Autodesk Inventor part; units mm, degrees
ref_plane "Plano de trabajo1" through (0, 5, -50) normal (1, 0, 0) x (0, 0, -1)
ref_plane "Plano de trabajo2" through (0, 15, 0) normal (0, -1, 0) x (1, 0, 0)
ref_plane "YZ Plane" through (0, 0, 0) normal (1, 0, 0) x (0, 1, 0)
sketch "Boceto1" plane through (0, 0, 0) normal (0, 1, 0) x (-1, 0, 0)
  line L0 (27.5, 50) -> (-27.5, 50)
  line L1 (-27.5, 50) -> (-27.5, -50)
  line L2 (-27.5, -50) -> (27.5, -50)
  line L3 (27.5, -50) -> (27.5, 50)
  line L4 (27.5, 50) -> (-27.5, -50) construction
  line L5 (-27.5, 50) -> (27.5, -50) construction
  point P0 (0, 0)
  dimension "d0" = 55
  dimension "d1" = 100
extrude "Extrusión1" add sketch "Boceto1" along normal blind 30
sketch "Boceto2" plane through (27.5, 0, -50) normal (0, 0, -1) x (-1, 0, 0)
  line L0 (22.5, 25) -> (32.5, 25)
  line L1 (32.5, 25) -> (32.5, 5)
  line L2 (32.5, 5) -> (22.5, 5)
  line L3 (22.5, 5) -> (22.5, 25)
  line L4 (22.5, 25) -> (32.5, 5) construction
  line L5 (32.5, 25) -> (22.5, 5) construction
  line L6 (0, 30) -> (55, 30)
  line L7 (0, 0) -> (0, 30)
  line L8 (55, 0) -> (55, 30)
  point P0 (27.5, 0)
  point P1 (27.5, 15)
  point P2 (27.5, 25)
  dimension "d4" = 10
  dimension "d5" = 20
  dimension "d6" = 5
  dimension "d7" = 22.5
  dimension "d24" = 22.5
extrude "Extrusión2" add sketch "Boceto2" along normal blind 10
sketch "Boceto3" plane through (-27.5, 0, 50) normal (0, 0, 1) x (1, 0, 0)
  circle A0 centre (27.5, 20) radius 5
  line L0 (0, 30) -> (55, 30)
  point P0 (27.5, 0)
  point P1 (27.5, 30)
  dimension "d10" = 10
  dimension "d11" = 10
extrude "Extrusión3" cut sketch "Boceto3" against normal blind 15
sketch "Boceto4" plane through (0, 30, 0) normal (0, 1, 0) x (1, 0, 0)
  line L0 (-20, 23) -> (20, 23)
  line L1 (20, 23) -> (20, -23)
  line L2 (20, -23) -> (-20, -23)
  line L3 (-20, -23) -> (-20, 23)
  line L4 (-20, 23) -> (20, -23) construction
  line L5 (20, 23) -> (-20, -23) construction
  point P0 (0, 0)
  dimension "d14" = 40
  dimension "d15" = 46
extrude "Extrusión4" cut sketch "Boceto4" against normal blind 20
ref_plane "Plano de trabajo1" through (0, 5, -50) normal (1, 0, 0) x (0, 0, -1)
sketch "Boceto5" plane through (0, 5, -50) normal (1, 0, 0) x (0, 0, -1)
  line L0 (7.5, 0) -> (0, -2.5)
  line L1 (0, -2.5) -> (0, 0)
  line L2 (0, 0) -> (7.5, 0)
  point P0 (-50, -5)
  point P1 (0, -5)
  point P2 (10, 0)
  dimension "d25" = 2.5
  dimension "d26" = 2.5
extrude "Extrusión5" add sketch "Boceto5" along normal mid plane 8
ref_plane "Plano de trabajo2" through (0, 15, 0) normal (0, -1, 0) x (1, 0, 0)
sketch "Boceto6" plane through (0, 15, 0) normal (0, -1, 0) x (1, 0, 0)
  line L0 (5, -50) -> (8, -50)
  line L1 (27.5, -50) -> (-27.5, -50)
  line L2 (5, -57) -> (8, -50)
  line L3 (4, -50) -> (5, -50)
  line L4 (5, -50) -> (5, -57)
  line L5 (0, -50.2371) -> (0, -56.5746)
  line L6 (-5, -50) -> (-8, -50)
  line L7 (-27.5, -50) -> (27.5, -50)
  line L8 (-5, -57) -> (-8, -50)
  line L9 (-4, -50) -> (-5, -50)
  line L10 (-5, -50) -> (-5, -57)
  point P0 (0, 0)
  point P1 (5, -60)
  point P2 (-5, -60)
  dimension "d29" = 3
  dimension "d30" = 3
extrude "Extrusión6" add sketch "Boceto6" along normal mid plane 8
sketch "Boceto7" plane through (27.5, 0, 50) normal (1, 0, 0) x (0, 0, -1)
  point P0 (50, 0)
ref_plane "Plano de trabajo4" through (-20, 30, -23) normal (0, 0, 1) x (1, 0, 0)
sketch "Boceto8" plane through (27.5, 0, 50) normal (1, 0, 0) x (0, 0, -1)
  line L0 (58, 22) -> (88, 22)
  circle A0 centre (83, 17) radius 1.75
  line L1 (63, 17) -> (83, 17)
  line L2 (88, 22) -> (88, 12)
  circle A1 centre (63, 17) radius 1.75
  line L3 (58, 12) -> (88, 22) construction
  line L4 (58, 22) -> (88, 12) construction
  line L5 (58, 12) -> (58, 22)
  line L6 (88, 12) -> (58, 12)
  line L7 (73, 30) -> (73, 10)
  line L8 (0, 30) -> (100, 30)
  point P0 (50, 0)
  point P1 (72.9522, 12.5553)
  point P2 (57.9522, 14.5161)
  point P3 (72.9522, 12.5553)
  point P4 (88, 17)
  dimension "d34" = 10
  dimension "d35" = 30
  dimension "d36" = 5
  dimension "d37" = 5
  dimension "d38" = 5
  dimension "d39" = 5
  dimension "d40" = 10
  dimension "d41" = 8
hole "Agujero1" at (27.5, 17, -13) at (27.5, 17, -33) direction (-1, 0, 0) diameter 3.5 end through all
properties part number "camera_support_2"
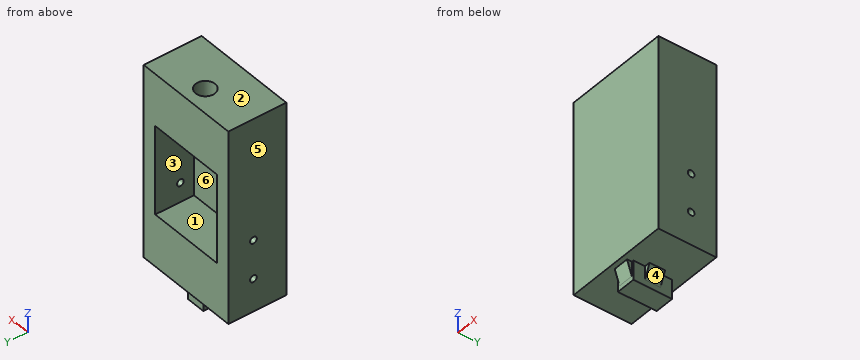
The model under review builds one solid part; all positions refer to its coordinate system, in mm. Face numbers are marked on the shaded views. A direction names the side the tool comes from. Give positions to 0.01 mm unless a question says otherwise; leave off trailing zeros. Write each loop counter-clockwise with the first axis right and the second up, starting at its lowest first coordinate (ties: lowest second). Pieces come first, ordered by that corner, then holes. Notation, with made-up numbers: M -13,86.5 L 23,86.5 A14 cw 23,101.5 Z; hole C 40,-34.5 d8. An arc over 180 degrees is marked long. Write item = value, one per line. Start each with the question number.
Q1. We need section C-C (x = 0). State the section outline as (y, z) points.
Q2. We need section B-B (y = 17). Give the number of separate pieces and of enclosed holes in the cut face, plus the area to 3 significant figures.
Q3. We need section A-A (z = -33). State the section outline as (x, y) points, plus the area to 3 significant figures.
Q4. Machinability: for the marked faces 1 and 2, which of the approach directions +Z, -Z, +X, -X, +Y, -Y give a long, thin tool a straight path to every point of the face, cutting with its end or side? Answer none if there is none.
Q5. Mouldability with a two-part tool opening along Z and no side actions: class the marked faces 3, 4, 5 and 6 as released by +Z, released by -Z, zero draft, split by the parting line, or undercut.
Q6. Clearance check with flat-ended pins moving along their axes: pin 1 (8 mm diameter, centred on x = -0.5, z = -57.5, fed in from -Y); pin 2 (2 mm diameter, centred on y = 17, z = -13, fed in from -X); pin 3 (1.5 mm diameter, centred on x = 3.5, z = -7.5, fed in from -Y); pin 4 (10 mm diameter, centred on x = 20.5, y = 24, fed in from -Z). State where each tip first meets the part, or that it passes through.
Q7. We need section D-D (x = 23). State the section outline as (y, z) points.
Q8. For line 1 (Z direction, x = 23.5, y = 17); line 2 (Z direction, x = -16.5, y = 24.25); line 3 (Z direction, x = 9.5, y = 17), list the stretches that pass through material, from the lowest coordinate up.
Result set:
q1.outline = M 0,-50 L 2.5,-50 L 5,-57.5 L 5,-60 L 25,-60 L 25,-50 L 30,-50 L 30,-23 L 10,-23 L 10,23 L 30,23 L 30,50 L 25,50 L 25,35 L 15,35 L 15,50 L 0,50 Z; hole C 17,-33 d3.5
q2.separate_pieces = 3
q2.enclosed_holes = 0
q2.area = 3,420 mm2
q3.outline = M -27.5,0 L 27.5,0 L 27.5,15.25 L -27.5,15.25 Z; M -27.5,18.75 L 27.5,18.75 L 27.5,30 L -27.5,30 Z
q3.area = 1,460 mm2
q4.face_1 = +Y
q4.face_2 = +Z, +X, -X, +Y, -Y
q5.face_3 = undercut
q5.face_4 = released by -Z
q5.face_5 = zero draft
q5.face_6 = undercut
q6.pin_1 = 3.67
q6.pin_2 = through
q6.pin_3 = 0
q6.pin_4 = -50
q7.outline = M 0,-50 L 30,-50 L 30,50 L 0,50 Z; hole C 17,-33 d3.5; hole C 17,-13 d3.5
q8.line_1 = -50 to -34.75, -31.25 to -14.75, -11.25 to 50
q8.line_2 = -50 to -23, 23 to 50
q8.line_3 = -50 to -34.75, -31.25 to -23, 23 to 50
